from build123d import *

# Parameters (mm, degrees)
BOSS_EXTRUDE1_DEPTH = 3.175
CUT_EXTRUDE1_REACH  = 5.175


with BuildPart() as part:
    # Sketch1 → Boss-Extrude1 (new body)
    with BuildSketch(Plane(origin=(0, 0, 0), x_dir=(1, 0, 0), z_dir=(0, 1, 0))):
        Polygon((0, 0), (10, 0), (10, 23), (8, 23), (8, 19.825), (6.5, 19.825), (6.5, 23), (3.5, 23), (3.5, 19.825), (2, 19.825), (2, 23), (0, 23), align=None)
    extrude(amount=BOSS_EXTRUDE1_DEPTH)

    # Sketch3 → Cut-Extrude1 (cut, up to next)
    with BuildSketch(Plane(origin=(0, 3.175, 0), x_dir=(1, 0, 0), z_dir=(0, 1, 0)), mode=Mode.PRIVATE) as cut_extrude1_sk1:
        with BuildLine():
            Line((3.605, 2), (6.385, 2))
            Line((6.385, 2), (6.385, 13.993552011))
            ThreePointArc((6.385, 13.993552011), (5.005949297, 18.717480034), (3.605, 14))
            Line((3.605, 14), (3.605, 2))
        make_face()
    cut_extrude1_tool1 = extrude(cut_extrude1_sk1.sketch, amount=-CUT_EXTRUDE1_REACH, mode=Mode.PRIVATE) & part.part
    add(cut_extrude1_tool1.solids().sort_by_distance((4.996868, 3.175, -11.078992))[0], mode=Mode.SUBTRACT)


solid = part.part
Source: CAD feature listing. Evaluate the final solid. Frame: model axes, mm. A direction names the side the tool comes from. Round coordinates to 2 decimals unless told otherwise and drop trailing zeros. Loops run counter-clockwise (first coordinate to the right, second up) from the corner with the lowest first, then second, coordinate; pieces in that order, holes last. Notation, with made-up numbers: (7, -14.75) -> (22, -14.75) arc R22 ccw to (22, 17.25) -> close; hole circle Ø2 at (-6.75, 28). An arc over 180 degrees is marked (long way). Answer as a JSON object with one key per item and string values. Group by question number.
Q1. Section query B-B (z = -21.5). Output: boundary loops of the cut face in (x, y) (3 decimals), plus the area to 3 significant figures.
Q2. Section query A-A (y = 0.45). Output: boundary loops of the cut face in (x, z) (3 decimals), plus the area to 3 significant figures.
Q3. Ray query, line 1 (X direction, y = 1.15, z = -20); line 2 (Z direction, x = 5, y = 2.55); line 3 (X direction, y = 0.1, z = -2.75) (3 decimals). Return the intervals inside material, ascending. Write a range as from..to.
Q4. Access query for faces 4 (the flat face through (3, 3.175, -12)), 5 (the flat face through (3, 2, -19.825)), 6 (the flat face through (5, 2, -2)). Directions: +Z, -Z, +X, -X, +Y, -Y. A direction counts if a zero-diameter tool reaches every point of the face in a straight line with its end or side. Return the directions, or none.
Q5. Mould query, pull axis X, two halves, no side actions, for faces 1 (the flat face through (3.5, 2, -21)), 2 (the flat face through (1, 2, -23)), 3 (the flat face through (0, 2, -12)). Classes: pulls with the +X half, pulls with the -X half, needs draft (parallel to the pull), parting line crosses it, or undercut.
Q6. Section query D-D (z = -11.5). Output: boundary loops of the cut face in (x, y) (3 decimals).
Q7. Section query C-C (x = 5). Output: boundary loops of the cut face in (y, z) (3 decimals).
Completed:
{
 "1": {"outline": "(0, 0) -> (2, 0) -> (2, 3.175) -> (0, 3.175) -> close; (3.5, 0) -> (6.5, 0) -> (6.5, 3.175) -> (3.5, 3.175) -> close; (8, 0) -> (10, 0) -> (10, 3.175) -> (8, 3.175) -> close", "area": "22.2 mm²"},
 "2": {"outline": "(0, -23) -> (2, -23) -> (2, -19.825) -> (3.5, -19.825) -> (3.5, -23) -> (6.5, -23) -> (6.5, -19.825) -> (8, -19.825) -> (8, -23) -> (10, -23) -> (10, 0) -> (0, 0) -> close; hole (3.605, -14) arc R2.565 ccw (long way) to (6.385, -13.994) -> (6.385, -2) -> (3.605, -2) -> close", "area": "167 mm²"},
 "3": {"line 1": "0..2, 3.5..6.5, 8..10", "line 2": "-23..-18.72, -2..0", "line 3": "0..3.605, 6.385..10"},
 "4": {"face 4": "+Z, -Z, +X, -X, +Y", "face 5": "-Z, +Y, -Y", "face 6": "+Y, -Y"},
 "5": {"face 1": "undercut", "face 2": "needs draft", "face 3": "pulls with the -X half"},
 "6": {"outline": "(0, 0) -> (3.605, 0) -> (3.605, 3.175) -> (0, 3.175) -> close; (6.385, 0) -> (10, 0) -> (10, 3.175) -> (6.385, 3.175) -> close"},
 "7": {"outline": "(0, -23) -> (3.175, -23) -> (3.175, -18.717) -> (0, -18.717) -> close; (0, -2) -> (3.175, -2) -> (3.175, 0) -> (0, 0) -> close"}
}
